Autodesk Inventor part; units mm, degrees
ref_plane "YZ Plane" through (0, 0, 0) normal (1, 0, 0) x (0, 1, 0)
ref_plane "XZ Plane" through (0, 0, 0) normal (0, 1, 0) x (-1, 0, 0)
ref_plane "XY Plane" through (0, 0, 0) normal (0, 0, 1) x (1, 0, 0)
sketch "Sketch1" plane through (0, 0, 0) normal (0, 1, 0) x (-1, 0, 0)
  line L0 (0, 0) -> (0, -12.7)
  line L1 (0, -12.7) -> (25.4, -12.7)
  line L2 (25.4, -12.7) -> (25.4, 12.7)
  line L3 (25.4, 12.7) -> (12.7, 12.7)
  line L4 (12.7, 12.7) -> (12.7, 0)
  line L5 (12.7, 0) -> (0, 0)
  arc A0 (6.35, 0) -> (6.35, -12.7) centre (6.35, -6.35) ccw
  dimension "d0" = 12.7
  dimension "d1" = 25.4
  dimension "d2" = 25.4
  dimension "d3" = 12.7
extrude "Extrusion1" add sketch "Sketch1" along normal blind 12.7 contours A0 L5 L4 L3 L2 L1
sketch "Sketch2" plane through (-25.4, 0, -12.7) normal (-1, 0, 0) x (0, 0, 1)
  line L0 (25.4, 0) -> (25.4, 12.7)
  point P0 (12.7, 0)
  point P1 (19.05, 6.35)
  point P2 (25.4, 6.35)
  dimension "d6" = 6.35
sketch "Sketch3" plane through (0, 0, -12.7) normal (0, 0, -1) x (-1, 0, 0)
  line L0 (0, 0) -> (0, 12.7)
  line L1 (12.7, 0) -> (12.7, 12.7)
  line L2 (0, 10.16) -> (12.7, 10.16)
  line L3 (12.7, 10.16) -> (12.7, 2.54)
  line L4 (12.7, 2.54) -> (0, 2.54)
  line L5 (0, 2.54) -> (0, 10.16)
  line L6 (25.4, 0) -> (25.4, 12.7)
  line L7 (12.7, 2.54) -> (25.4, 2.54)
  line L8 (25.4, 2.54) -> (25.4, 10.16)
  line L9 (25.4, 10.16) -> (12.7, 10.16)
  line L10 (12.7, 10.16) -> (12.7, 2.54)
  point P0 (12.7, 6.35)
  point P1 (0, 2.54)
  dimension "d15" = 7.62
extrude "Extrusion2" cut sketch "Sketch3" against normal blind 12.7
sketch "Sketch4" plane through (0, 12.7, 0) normal (0, 1, 0) x (1, 0, 0)
  line L0 (0, 0) -> (0, 12.7)
  line L1 (-12.7, 0) -> (0, 0)
  line L2 (-12.7, -12.7) -> (-12.7, 0)
  line L3 (-12.7, 0) -> (-12.7, 12.7)
  point P0 (-6.35, 6.35)
  point P1 (0, 6.35)
  point P2 (-6.35, 0)
  point P3 (-19.05, 6.35)
hole "Hole2" at (-6.35, 12.7, -6.35) at (-19.05, 12.7, -6.35) direction (0, -1, 0) diameter 6.7564 depth 12.7 tip angle 118
hole "Hole3" at (-25.4, 6.35, 6.35) direction (1, 0, 0) diameter 6.7564 depth 12.7 tip angle 118
ref_plane "Work Plane1" through (-6.35, 12.7, 0) normal (1, 0, 0) x (0, 0, -1)
fillet "Fillet1" radius 5 2 edges at (-25.4, 11.43, -12.7) (-25.4, 1.27, -12.7)
properties part number "Locker"
Input: part model. Units: mm. Frame: model coordinates. A direction names the side the tool comes from. Coordinates: 2 decimals unless noted, no trailing zeros. Loops run counter-clockwise (first coordinate to the right, second up) from the corner with the lowest first, then second, coordinate; pieces in that order, holes last. Notation, with made-up numbers: (45.25, 76.25) -> (75.25, 76.25) arc R27 ccw to (75.25, 103.25) -> close; hole circle Ø6 at (-9.75, 7). An arc over 180 degrees is marked (long way). One line per item, written item: value.
(1) Ray query, line 1 along X through (y, z) = (0.8, -6.35); line 2 along Y through (x, z) = (-23, -10.75); line 3 along Z through (x, y) = (-19.05, 1). Return the intervals inside material, ascending.
Answer below:
line 1: x = -25.4 to -22.43, -15.67 to -9.73, -2.97 to 0
line 2: y = 0 to 2.54, 10.16 to 12.7
line 3: z = -12.7 to -9.73, -2.97 to 12.7
(2) Draft query along Z for faces 1 (the face through (-16.053, 11.412, -4.791)), 2 (the face through (-12.7, 3, 4)), 3 (the face through (0, 11.4, -6.5)). Return one class per face: pulls with the +Z half, pulls with the -Z half, needs draft (parallel to the pull), parting line crosses it, or undercut.
Answer below:
face 1: undercut
face 2: needs draft
face 3: parting line crosses it
(3) Pin query (flat end, axial travel): pin 1 Ø1.3 at (x, y) = (-8.5, 2) entering from +Z; pin 2 Ø1 at (y, z) = (1.5, -8.5) entering from -X. Return the tip coordinate at first contact, or that it passes through.
Answer below:
pin 1: stops at z = 0
pin 2: stops at x = -25.39
(4) Cut plane A-A (x = -19.05). Output: boundary loops of the cut face in (y, z), then the cut area to 3 significant figures.
Answer below:
outline: (0, -12.7) -> (2.54, -12.7) -> (2.54, -9.73) -> (0, -9.73) -> close; (0, -2.97) -> (2.54, -2.97) -> (2.54, 0) -> (10.16, 0) -> (10.16, -2.97) -> (12.7, -2.97) -> (12.7, 12.7) -> (0, 12.7) -> close; (10.16, -12.7) -> (12.7, -12.7) -> (12.7, -9.73) -> (10.16, -9.73) -> close; hole circle Ø6.76 at (6.35, 6.35)
area: 156 mm2
(5) Cut plane B-B (z = -6.35). Output: boundary loops of the cut face in (x, y).
Answer below:
outline: (-25.4, 0) -> (-22.43, 0) -> (-22.43, 2.54) -> (-25.4, 2.54) -> close; (-25.4, 10.16) -> (-22.43, 10.16) -> (-22.43, 12.7) -> (-25.4, 12.7) -> close; (-15.67, 0) -> (-9.73, 0) -> (-9.73, 2.54) -> (-15.67, 2.54) -> close; (-15.67, 10.16) -> (-9.73, 10.16) -> (-9.73, 12.7) -> (-15.67, 12.7) -> close; (-2.97, 0) -> (0, 0) -> (0, 2.54) -> (-2.97, 2.54) -> close; (-2.97, 10.16) -> (0, 10.16) -> (0, 12.7) -> (-2.97, 12.7) -> close
(6) Set-up query: faces 4 (the face through (-10, 11, 0)), 5 (the face through (-19, 6, 0)), 6 (the face through (-7.365, 1.252, -3.128)). Return all of +Z, -Z, +X, -X, +Y, -Y with unobstructed straight access to the full face (end or side cutting, diameter ignored); none if empty.
Answer below:
face 4: +Z, +X, +Y, -Y
face 5: -Z, +X, -X
face 6: +Y, -Y
(7) Cut plane C-C (y = 6.35). Output: boundary loops of the cut face in (x, z).
Answer below:
outline: (-25.4, 0) -> (-12.7, 0) -> (-12.7, 2.97) -> (-25.4, 2.97) -> close; (-25.4, 9.73) -> (-12.7, 9.73) -> (-12.7, 12.7) -> (-25.4, 12.7) -> close
